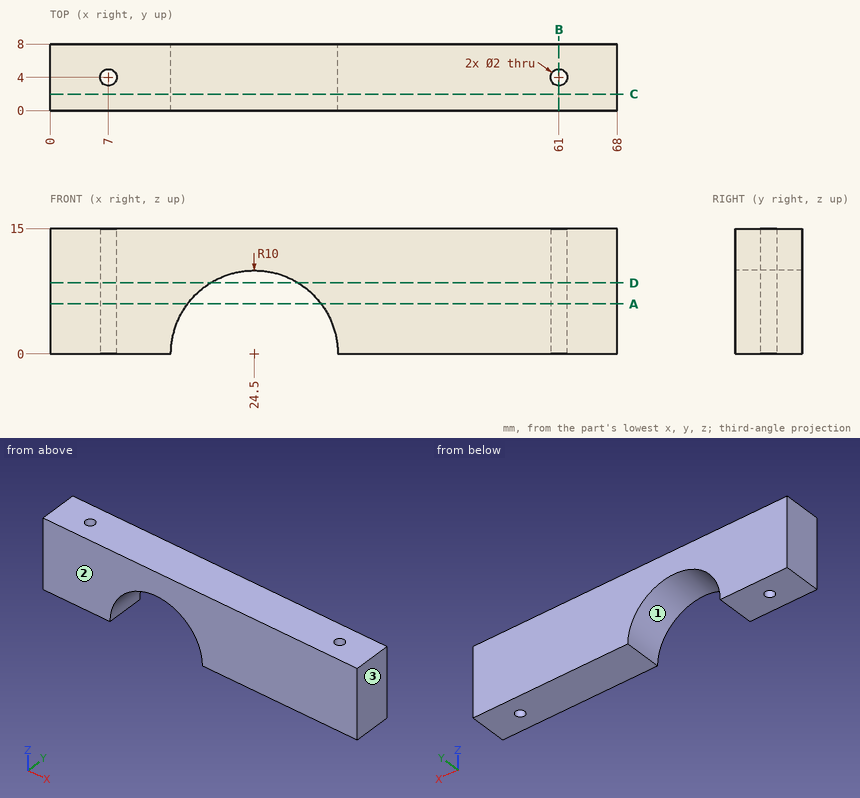
The drawing under review shows one solid part. Ordinate dimensions are in mm from its lowest x, y, z. Coordinates: 2 decimals unless noted, no trailing zeros. Loops run counter-clockwise (first coordinate to the right, second up) from the corner with the lowest first, then second, coordinate; pieces in that order, holes last. Notation, with made-up numbers: M -3.75,24 L 42.25,24 A21 ccw 42.25,37 Z; hole C 34,34.5 d8. An arc over 180 degrees is marked long. Use one line per item in the form item = value.
(1) Consider section A-A (z = 6). Write out the cut boundary in (x, y).
Return value:
outline = M 0,0 L 16.5,0 L 16.5,8 L 0,8 Z; M 32.5,0 L 68,0 L 68,8 L 32.5,8 Z; hole C 7,4 d2; hole C 61,4 d2
(2) Clearance check with a flat-ended pin moving along its axis: P1, Ø3, axis at x = 7, y = 4, coming from the +Z side. State where the tip first meets the part, or that it passes through.
Return value:
P1 = 15
(3) Draft analysis for pull direction X (two halves, no side actions). For the marked faces 1, 2 and 3, state which applies: pulls with the +X half, pulls with the -X half, needs draft (parallel to the pull), parting line crosses it, or undercut.
Return value:
face_1 = undercut
face_2 = needs draft
face_3 = pulls with the +X half
(4) Consider section C-C (y = 2). Write out the cut boundary in (x, z), and give its area (3 significant figures).
Return value:
outline = M 0,0 L 14.5,0 A10 cw 34.5,0 L 68,0 L 68,15 L 0,15 Z
area = 863 mm2
(5) For line 1 along X through (y, z) = (4, 11); line 2 along Y through (x, z) = (7, 4.5); line 3 along X through (y, z) = (3.5, 12.5), list the stretches that pass through material, from the lowest coordinate up. Write a range as from..to.
Return value:
line_1 = 0..6, 8..60, 62..68
line_2 = 0..3, 5..8
line_3 = 0..6.13, 7.87..60.13, 61.87..68
(6) Consider section B-B (x = 61). Write out the cut boundary in (y, z), and give its area (3 significant figures).
Return value:
outline = M 0,0 L 3,0 L 3,15 L 0,15 Z; M 5,0 L 8,0 L 8,15 L 5,15 Z
area = 90.0 mm2
(7) Consider section D-D (z = 8.5). Write out the cut boundary in (x, y).
Return value:
outline = M 0,0 L 19.23,0 L 19.23,8 L 0,8 Z; M 29.77,0 L 68,0 L 68,8 L 29.77,8 Z; hole C 7,4 d2; hole C 61,4 d2
